from build123d import *

# Parameters (mm, degrees)
SKETCH_1_R      = 5
EXTRUDE_1_DEPTH = 90
SKETCH_2_W      = 6.5
SKETCH_2_H      = 4
EXTRUDE_2_DEPTH = 20
CHAMFER_1_SIZE  = 2


with BuildPart() as part:
    # 草图1 → 凸台-拉伸1 (new body)
    with BuildSketch(Plane.XY):
        with Locations(Location((0, 0, 0), (0, 0, 180))):
            Circle(SKETCH_1_R)
    extrude(amount=EXTRUDE_1_DEPTH)

    # 草图2 → 凸台-拉伸2 (add)
    with BuildSketch(Plane.XY.offset(90)):
        with Locations((-3.25, 0)):
            Rectangle(SKETCH_2_W, SKETCH_2_H)
    extrude(amount=-EXTRUDE_2_DEPTH)

    # 倒角1
    chamfer_1_edges = [part.edges().sort_by_distance(p)[0] for p in [
        (5, 0, 90),
    ]]
    chamfer(chamfer_1_edges, length=CHAMFER_1_SIZE)


solid = part.part
The model under review builds one solid part; all positions refer to its coordinate system, in mm. A direction names the side the tool comes from. Give positions to 0.01 mm unless a question says otherwise; leave off trailing zeros. Write each loop counter-clockwise with the first axis right and the second up, starting at its lowest first coordinate (ties: lowest second). Pieces come first, ordered by that corner, then holes.
1. Wall thickness on L1, parallel to Y at x = -0.25, z = 57; L2, parallel to Y at x = -4.75, z = 77; L3, parallel to X at y = 4, z = 62: over which ranges is each line inside the solid? List them lowest first.
2. Add section B-B, the plane z = 38. Write out the cut boundary in (x, y), plus the area to 3 significant figures.
3. Add section A-A, the plane y = 0. Write out the cut boundary in (x, z).
4. Tool access review of faces 1 (the flat face through (0, 0, 0)), 2 (the cylindrical face through (5, 0, 43)): name each direction out of +Z, -Z, +X, -X, +Y, -Y from which nothing blocks a thin tool from reaching the whole face with its end or side.
5. For P1, Ø3.5, axis at x = -5.5, z = 78, coming from the +Y side; P2, Ø3, axis at x = 1, y = 3, coming from the +Z side; P3, Ø2, axis at y = 2.5, z = 23.5, coming from the -X side; P4, Ø1.3, axis at x = -4.5, z = 76.5, coming from the -Y side, all flat-tipped, find the tip position at first contact; note any pin that passes through.
Worked answers:
1. L1: y = -4.99 to 4.99
1. L2: y = -2 to 2
1. L3: x = -3 to 3
2. outline: circle Ø10 at (0, 0)
2. area: 78.5 mm2
3. outline: (-6.5, 70) - (-5, 70) - (-5, 0) - (5, 0) - (5, 88) - (3, 90) - (-6.5, 90) - close
4. face 1: -Z, +X, -X, +Y, -Y
4. face 2: -Z
5. P1: stops at y = 3.31
5. P2: stops at z = 90
5. P3: stops at x = -4.77
5. P4: stops at y = -3.19
